from build123d import *

# Parameters (mm, degrees)
F1_W     = 8
F1_H     = 58
F2_DEPTH = 8
F3_W     = 8
F3_H     = 8
F4_DEPTH = 21
F5_R     = 1.75
F6_DEPTH = 30
F7_W     = 6.4
F7_H     = 3
F8_DEPTH = 25
F9_DEPTH = 30


# Not quite as in the source:
# - a feature names something its author has since deleted; it is built from what else it names


with BuildPart() as f2:
    # F1 (on Top) → F2 (new body)
    with BuildSketch(Plane.XY):
        Rectangle(F1_W, F1_H)
    extrude(amount=F2_DEPTH)

    # F3 (on face) → F4 (join)
    with BuildSketch(Plane.XY.offset(8)):
        with Locations((0, 25)):
            Rectangle(F3_W, F3_H)
        with Locations((0, -25)):
            Rectangle(F3_W, F3_H)
    extrude(amount=F4_DEPTH)

    # F5 (on face) → F6 (cut)
    with BuildSketch(Plane.XY.offset(29)):
        with Locations((0, 25)):
            Circle(F5_R)
    extrude(amount=-F6_DEPTH, mode=Mode.SUBTRACT)

    # F7 (on face) → F8 (cut)
    with BuildSketch(Plane(origin=(-4, 0, 0), x_dir=(0, -1, 0), z_dir=(-1, 0, 0))):
        with Locations((-25, 25.5)):
            Rectangle(F7_W, F7_H)
        with Locations((25, 25.5)):
            Rectangle(F7_W, F7_H)
    extrude(amount=-F8_DEPTH, mode=Mode.SUBTRACT)

    # F5 (on face) → F9 (cut)
    with BuildSketch(Plane.XY.offset(29)):
        with Locations((0, 25)):
            Circle(F5_R)
        with Locations((0, -25)):
            Circle(F5_R)
    extrude(amount=-F9_DEPTH, mode=Mode.SUBTRACT)


solid = f2.part
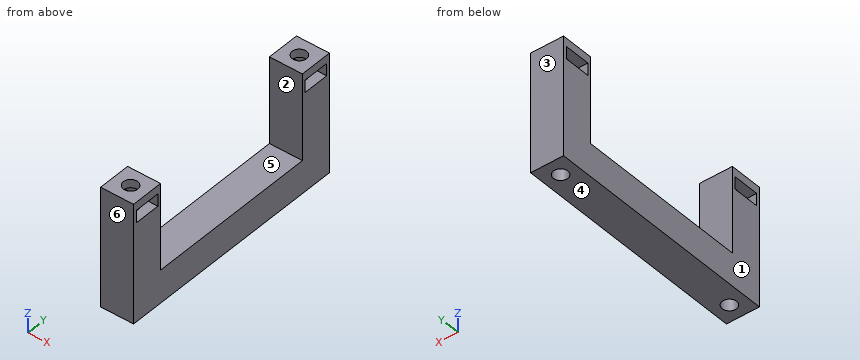
Geometry: final body of the model. Coordinates: model frame, mm. Face numbers are marked on the shaded views. A direction names the side the tool comes from. Give positions to 0.01 mm unless a question says otherwise; leave off trailing zeros. Loops run counter-clockwise (first coordinate to the right, second up) from the corner with the lowest first, then second, coordinate; pieces in that order, holes last. Notation, with made-up numbers: (-26.5, 72) - (32.5, 72) arc R18 ccw to (32.5, 91) - close; hole circle Ø7 at (28.25, -31.5). An arc over 180 degrees is marked (long way). Answer as CSV lines item,"result". Start each with the question number.
1. Section A-A, the plane z = 20. Return loops of the section in (x, y).
2. Section C-C, the plane y = -25. Return loops of the section in (x, z), plus the area to 3 significant figures.
3. Reachability of the marked faces 1 and 2 from +Z, -Z, +X, -X, +Y, -Y: full face, straight path, thin tool, end or side. Return the list, or none.
4. Section D-D, the plane z = 3. Return loops of the section in (x, y), plus the area to 3 significant figures.
5. Section B-B, the plane x = 0. Give the number of separate pieces and of enclosed holes in the cut face, plus the area to 3 significant figures.
6. Draft query along Y for the marked faces 3, 4, 5 and 6. Return one class per face: released by +Y, released by -Y, zero draft, split by the parting line, or undercut.
7. Ray query, L1, parallel to Y at x = 0, z = 27.45; L2, parallel to Y at x = 0, z = 6; L3, parallel to Z at x = -1.75, y = -23. Return the intervals inside material, ascending.
8. Pin query (flat end, axial travel): P1, Ø4, axis at x = 0, y = -25, coming from the +Z side. Return the tip coordinate at first contact, or that it passes through.
Answers:
1,outline,"(-4, -29) - (4, -29) - (4, -21) - (-4, -21) - close; (-4, 21) - (4, 21) - (4, 29) - (-4, 29) - close; hole circle Ø3.5 at (0, -25); hole circle Ø3.5 at (0, 25)"
2,outline,"(-4, 0) - (-1.75, 0) - (-1.75, 24) - (-4, 24) - close; (-4, 27) - (-1.75, 27) - (-1.75, 29) - (-4, 29) - close; (1.75, 0) - (4, 0) - (4, 24) - (1.75, 24) - close; (1.75, 27) - (4, 27) - (4, 29) - (1.75, 29) - close"
2,area,"117 mm2"
3,face 1,"+Z, -Z, -X, +Y, -Y"
3,face 2,"+Z, +X, -X"
4,outline,"(-4, -29) - (4, -29) - (4, 29) - (-4, 29) - close; hole circle Ø3.5 at (0, -25); hole circle Ø3.5 at (0, 25)"
4,area,"445 mm2"
5,separate pieces,"3"
5,enclosed holes,"0"
5,area,"580 mm2"
6,face 3,"released by +Y"
6,face 4,"zero draft"
6,face 5,"undercut"
6,face 6,"released by -Y"
7,L1,"y = -29 to -26.75, -23.25 to -21, 21 to 23.25, 26.75 to 29"
7,L2,"y = -29 to -26.75, -23.25 to 23.25, 26.75 to 29"
7,L3,"z = 0 to 24, 27 to 29"
8,P1,"stops at z = 29"
